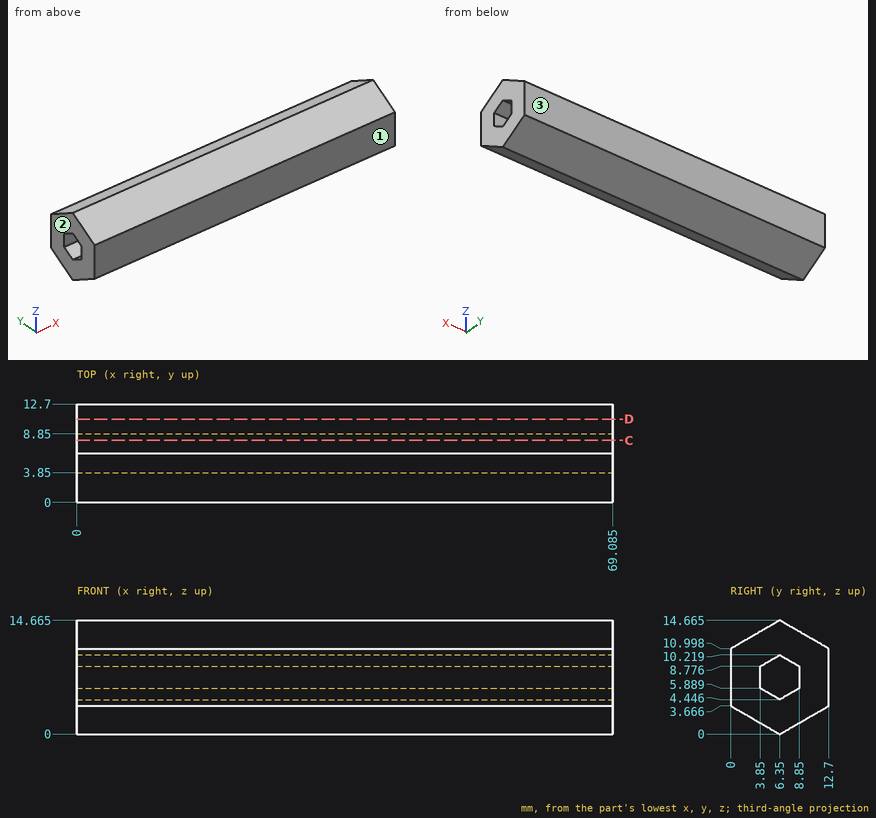
Answer from the drawing. Dimensions are ordinates in mm from the lowest x, y and z of the part. Round coordinates to 2 decimals unless told otherwise and drop trailing zeros. Order: outer loops, then holes, each group sorted by start corner. A loop starts at its lowest first (then second) coordinate and runs counter-clockwise, first axis right, second up. Notation, with made-up numbers: (-35, 51) -> (21, 51) arc R20 cw to (21, 63) -> close; hole circle Ø11 at (-13.75, 81.25). An arc over 180 degrees is marked (long way). Answer as CSV lines item,"result".
Q1. A cutting plane is placed at D-D on y = 10.75. Determine the outline of the cut face in (x, z) (1 decimal).
Computed values:
outline,"(0, 2.5) -> (69.1, 2.5) -> (69.1, 12.1) -> (0, 12.1) -> close"
Q2. For a pull along Y with two mould halves and no side action, classify the marked faces 1, 2 and 3 as +Y half, -Y half, draft (parallel to the pull), parting line (faces both ways), or undercut.
Computed values:
face 1,"-Y half"
face 2,"draft"
face 3,"+Y half"
Q3. Consider line 1 (Y direction, x = 63, z = 6.5); line 2 (Z direction, x = 23, y = 6.75) (1 decimal); line 3 (Y direction, x = 50, z = 5.5) (1 decimal). Determine where each line is inside the solid, lowest interval first. Write a range as from..to.
Computed values:
line 1,"y = 0..3.85, 8.85..12.7"
line 2,"z = 0.2..4.7, 10..14.4"
line 3,"y = 0..4.5, 8.2..12.7"
Q4. Given pin 1 (1 mm diameter, centred on x = 50.5, z = 13, fed in from +Y); pin 2 (6 mm diameter, centred on x = 55, y = 7, fed in from +Z) (1 decimal); pin 3 (6 mm diameter, centred on x = 23.5, y = 11, fed in from -Z); pin 4 (4 mm diameter, centred on y = 4.5, z = 12.5, fed in from -X), each flat-ended and moving along its own axis, determine where each tip first touches the part or whether it passes through.
Computed values:
pin 1,"stops at y = 10.1"
pin 2,"stops at z = 14.7"
pin 3,"stops at z = 0.95"
pin 4,"stops at x = 0"
Q5. A cutting plane is placed at C-C on y = 8. Determine the outline of the cut face in (x, z) (1 decimal).
Computed values:
outline,"(0, 1) -> (69.1, 1) -> (69.1, 5.4) -> (0, 5.4) -> close; (0, 9.3) -> (69.1, 9.3) -> (69.1, 13.7) -> (0, 13.7) -> close"
